from build123d import *

# Parameters (mm, degrees)
STOCK_HORN_DRIVE_FLANGE_START                 = 41
STOCK_HORN_DRIVE_FLANGE_PROFILE_R             = 13
STOCK_HORN_DRIVE_FLANGE_PROFILE_R_2           = 4.05
STOCK_HORN_DRIVE_FLANGE_DEPTH                 = 3
D_COUPLING_RING_START                         = 44
D_COUPLING_RING_PROFILE_R                     = 7
D_COUPLING_RING_PROFILE_R_2                   = 4.05
D_COUPLING_RING_DEPTH                         = 4
D_KEY_LAND_START                              = 44
D_KEY_LAND_PROFILE_W                          = 2.9
D_KEY_LAND_PROFILE_H                          = 4.8
D_KEY_LAND_DEPTH                              = 4
YAW_POSITIVE_RETENTION_CROSSBOLT_START        = -10
YAW_POSITIVE_RETENTION_CROSSBOLT_PROFILE_R    = 1.1
YAW_POSITIVE_RETENTION_CROSSBOLT_DEPTH        = 62.400389104
CROSSBOLT_FLAT_SEAT_CUT_12_START              = -12
CROSSBOLT_FLAT_SEAT_12_R                      = 2.75
CROSSBOLT_FLAT_SEAT_CUT_12_DEPTH              = 6
CROSSBOLT_FLAT_SEAT_CUT_6_START               = 6
CROSSBOLT_FLAT_SEAT_6_R                       = 2.75
CROSSBOLT_FLAT_SEAT_CUT_6_DEPTH               = 6
SG90_SPLINE_SOCKET_BOSS_OD12_START            = 37.3
SG90_SPLINE_SOCKET_BOSS_PROFILE_R             = 6
SG90_SPLINE_SOCKET_BOSS_OD12_DEPTH            = 3.7
SG90_SPLINE_PRESS_SOCKET_D4P85_DEPTH2P5_START = 37.3
SG90_SPLINE_PRESS_SOCKET_D4P85_DEPTH_2_R      = 2.425
SG90_SPLINE_PRESS_SOCKET_D4P85_DEPTH2P5_DEPTH = 2.5
SG90_CENTRE_SCREW_CLEARANCE_D2P4_START        = 39.8
SG90_CENTRE_SCREW_CLEARANCE_D2P4_PROFILE_R    = 1.2
SG90_CENTRE_SCREW_CLEARANCE_D2P4_DEPTH        = 1.2
CROSSBOLT_AXIAL_FLOAT_CLEARANCE_D2P8_START    = -10
CROSSBOLT_AXIAL_FLOAT_CLEARANCE_D2P8_PRO_R    = 1.4
CROSSBOLT_AXIAL_FLOAT_CLEARANCE_D2P8_DEPTH    = 62.400389197


with BuildPart() as part:
    # Stock_horn_drive_flange_profile → Stock_horn_drive_flange (new body)
    with BuildSketch(Plane(origin=(0, 0, 0), x_dir=(1, 0, 0), z_dir=(0, 1, 0)).offset(STOCK_HORN_DRIVE_FLANGE_START)):
        with Locations(Location((0, 0, 0), (0, 0, 270))):
            Circle(STOCK_HORN_DRIVE_FLANGE_PROFILE_R)
        with Locations(Location((0, 0, 0), (0, 0, 270))):
            Circle(STOCK_HORN_DRIVE_FLANGE_PROFILE_R_2, mode=Mode.SUBTRACT)
    extrude(amount=STOCK_HORN_DRIVE_FLANGE_DEPTH)

    # D_coupling_ring_profile → D_coupling_ring (add)
    with BuildSketch(Plane(origin=(0, 0, 0), x_dir=(1, 0, 0), z_dir=(0, 1, 0)).offset(D_COUPLING_RING_START)):
        with Locations(Location((0, 0, 0), (0, 0, 270))):
            Circle(D_COUPLING_RING_PROFILE_R)
        with Locations(Location((0, 0, 0), (0, 0, 270))):
            Circle(D_COUPLING_RING_PROFILE_R_2, mode=Mode.SUBTRACT)
    extrude(amount=D_COUPLING_RING_DEPTH)

    # D_key_land_profile → D_key_land (add)
    with BuildSketch(Plane(origin=(0, 0, 0), x_dir=(1, 0, 0), z_dir=(0, 1, 0)).offset(D_KEY_LAND_START)):
        with Locations((4.55, 0)):
            Rectangle(D_KEY_LAND_PROFILE_W, D_KEY_LAND_PROFILE_H)
    extrude(amount=D_KEY_LAND_DEPTH)

    # Yaw_positive_retention_crossbolt_profile → Yaw_positive_retention_crossbolt (cut, through all)
    with BuildSketch(Plane(origin=(0, 0, 0), x_dir=(0, 0, -1), z_dir=(1, 0, 0)).offset(YAW_POSITIVE_RETENTION_CROSSBOLT_START)):
        with Locations(Location((0, 45.5, 0), (0, 0, 180))):
            Circle(YAW_POSITIVE_RETENTION_CROSSBOLT_PROFILE_R)
    extrude(amount=YAW_POSITIVE_RETENTION_CROSSBOLT_DEPTH, mode=Mode.SUBTRACT)

    # Crossbolt_flat_seat_-12 → Crossbolt_flat_seat_cut_-12 (cut)
    with BuildSketch(Plane(origin=(0, 0, 0), x_dir=(0, 0, -1), z_dir=(1, 0, 0)).offset(CROSSBOLT_FLAT_SEAT_CUT_12_START)):
        with Locations((0, 45.5)):
            Circle(CROSSBOLT_FLAT_SEAT_12_R)
    extrude(amount=CROSSBOLT_FLAT_SEAT_CUT_12_DEPTH, mode=Mode.SUBTRACT)

    # Crossbolt_flat_seat_6 → Crossbolt_flat_seat_cut_6 (cut)
    with BuildSketch(Plane(origin=(0, 0, 0), x_dir=(0, 0, -1), z_dir=(1, 0, 0)).offset(CROSSBOLT_FLAT_SEAT_CUT_6_START)):
        with Locations((0, 45.5)):
            Circle(CROSSBOLT_FLAT_SEAT_6_R)
    extrude(amount=CROSSBOLT_FLAT_SEAT_CUT_6_DEPTH, mode=Mode.SUBTRACT)

    # SG90_spline_socket_boss_profile → SG90_spline_socket_boss_OD12 (add)
    with BuildSketch(Plane(origin=(0, 0, 0), x_dir=(1, 0, 0), z_dir=(0, 1, 0)).offset(SG90_SPLINE_SOCKET_BOSS_OD12_START)):
        with Locations(Location((0, 0, 0), (0, 0, 270))):
            Circle(SG90_SPLINE_SOCKET_BOSS_PROFILE_R)
    extrude(amount=SG90_SPLINE_SOCKET_BOSS_OD12_DEPTH)

    # SG90_spline_press_socket_D4p85_depth 2 → SG90_spline_press_socket_D4p85_depth2p5 (cut)
    with BuildSketch(Plane(origin=(0, 0, 0), x_dir=(1, 0, 0), z_dir=(0, 1, 0)).offset(SG90_SPLINE_PRESS_SOCKET_D4P85_DEPTH2P5_START)):
        with Locations(Location((0, 0, 0), (0, 0, 270))):
            Circle(SG90_SPLINE_PRESS_SOCKET_D4P85_DEPTH_2_R)
    extrude(amount=SG90_SPLINE_PRESS_SOCKET_D4P85_DEPTH2P5_DEPTH, mode=Mode.SUBTRACT)

    # SG90_centre_screw_clearance_D2p4_profile → SG90_centre_screw_clearance_D2p4 (cut)
    with BuildSketch(Plane(origin=(0, 0, 0), x_dir=(1, 0, 0), z_dir=(0, 1, 0)).offset(SG90_CENTRE_SCREW_CLEARANCE_D2P4_START)):
        with Locations(Location((0, 0, 0), (0, 0, 270))):
            Circle(SG90_CENTRE_SCREW_CLEARANCE_D2P4_PROFILE_R)
    extrude(amount=SG90_CENTRE_SCREW_CLEARANCE_D2P4_DEPTH, mode=Mode.SUBTRACT)

    # Crossbolt_axial_float_clearance_D2p8_profile → Crossbolt_axial_float_clearance_D2p8 (cut, through all)
    with BuildSketch(Plane(origin=(0, 0, 0), x_dir=(0, 0, -1), z_dir=(1, 0, 0)).offset(CROSSBOLT_AXIAL_FLOAT_CLEARANCE_D2P8_START)):
        with Locations((0, 45.5)):
            Circle(CROSSBOLT_AXIAL_FLOAT_CLEARANCE_D2P8_PRO_R)
    extrude(amount=CROSSBOLT_AXIAL_FLOAT_CLEARANCE_D2P8_DEPTH, mode=Mode.SUBTRACT)


solid = part.part
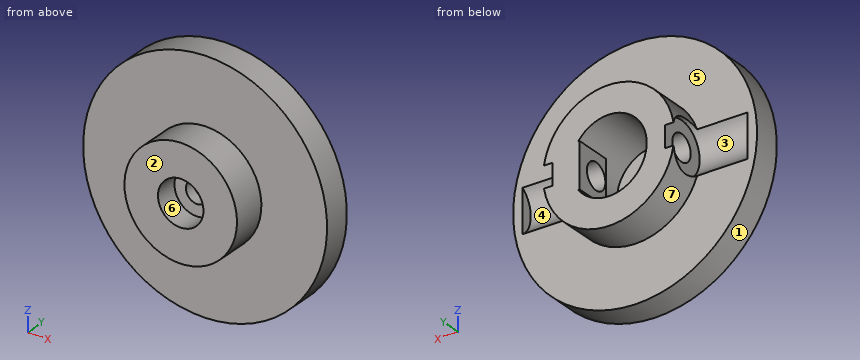
CAD build for the part. Positions are in the model's coordinates, mm. Face numbers are marked on the shaded views. A direction names the side the tool comes from. Give positions to 0.01 mm unless a question says otherwise; leave off trailing zeros. Loops run counter-clockwise (first coordinate to the right, second up) from the corner with the lowest first, then second, coordinate; pieces in that order, holes last. Notation, with made-up numbers: M -19,2.5 L 37,2.5 A26 cw 37,40.5 Z; hole C -21.75,24.25 d8. An arc over 180 degrees is marked long. One line per question, with ' | ' between items. Start each with the question number.
1. 3-axis set-ups, long thin cutter, end or side, ignore diameter. For the marked faces 4, 5, 6 and 7: which of +Z, -Z, +X, -X, +Y, -Y reach the whole face in a straight line?
2. Probe L1, parallel to X at y = 38.05, z = 0 (3 decimals); L2, parallel to Y at x = -4.75, z = 0; L3, parallel to Z at x = -1, y = 40.25. List the from-to ranges inside material, lowest first. Write a range as from..to.
3. Flat gauge pins, fed straight in: pin 1 (1.5 mm diameter, centred on x = 9, z = -10, fed in from -Y); pin 2 (1.5 mm diameter, centred on x = -10, y = 42, fed in from +Z); pin 3 (2.5 mm diameter, centred on y = 45, z = 0, fed in from -X); pin 4 (2.5 mm diameter, centred on x = 1.5, z = 1.5, fed in from +Y). Where does each tip first touch, or does it go through?
4. Saw through at B-B on y = 45.5. Give the cut face in (x, z), plus the area to 3 significant figures.
5. Two-plate mould, pull along X, no slides. Class the marked faces 1, 2 and 3: pulls with the +X half, pulls with the -X half, needs draft (parallel to the pull), parting line crosses it, or undercut.
6. Saw through at A-A on x = 0. Give the cut face in (y, z) (3 decimals).
7. Saw through at D-D on y = 42. Give the cut face in (x, z), plus the area to 3 significant figures.
8. Saw through at C-C on z = 0. State how many separate pieces and enclosed holes the cut face has, plus the area to 3 significant figures.
Result sheet:
1) face 4: none | face 5: +Y | face 6: -Y | face 7: -Z, +Y
2) L1: x = -6..-2.425, 2.425..6 | L2: y = 37.3..44.1, 46.9..48 | L3: z = -5.92..-0.66, 0.66..5.92
3) pin 1: stops at y = 41 | pin 2: stops at z = 9.13 | pin 3: stops at x = -13 | pin 4: stops at y = 41
4) outline: M -6.44,-2.75 A7 ccw 6.44,-2.75 L 6,-2.75 L 6,-1.4 L 3.1,-1.4 L 3.1,-2.4 L 3.26,-2.4 A4.05 cw -3.8,-1.4 L -6,-1.4 L -6,-2.75 Z; M -6.44,2.75 L -6,2.75 L -6,1.4 L -3.8,1.4 A4.05 cw 3.26,2.4 L 3.1,2.4 L 3.1,1.4 L 6,1.4 L 6,2.75 L 6.44,2.75 A7 ccw Z | area: 83.0 mm^2
5) face 1: parting line crosses it | face 2: needs draft | face 3: undercut
6) outline: M 37.3,-6 L 41,-6 L 41,-13 L 44,-13 L 44,-7 L 48,-7 L 48,-4.05 L 41,-4.05 L 41,-1.2 L 39.8,-1.2 L 39.8,-2.425 L 37.3,-2.425 Z; M 37.3,2.425 L 39.8,2.425 L 39.8,1.2 L 41,1.2 L 41,4.05 L 48,4.05 L 48,7 L 44,7 L 44,13 L 41,13 L 41,6 L 37.3,6 Z
7) outline: C 0,0 d26; hole C 0,0 d8.1 | area: 479 mm^2
8) separate pieces: 4 | enclosed holes: 0 | area: 73.9 mm^2
